from build123d import *

# Parameters (mm, degrees)
EXTRUDE_1_DEPTH     = 35
SKETCH_2_R          = 1.75
CUT_EXTRUDE_1_DEPTH = 40.39586793
SKETCH_3_W          = 0.8
SKETCH_3_H          = 10
EXTRUDE_2_DEPTH     = 35
SKETCH_4_R          = 2.7
CUT_EXTRUDE_2_DEPTH = 40.395868074


with BuildPart() as part:
    # Эскиз1 → Бобышка-Вытянуть1 (new body)
    with BuildSketch(Plane(origin=(0, 0, 0), x_dir=(1, 0, 0), z_dir=(0, 1, 0))):
        with BuildLine():
            Line((-4.558992206, 17.5), (0, 17.5))
            Line((0, 17.5), (0, -17.5))
            Line((0, -17.5), (-4.558992206, -17.5))
            ThreePointArc((-4.558992206, -17.5), (-3, 0), (-4.558992206, 17.5))
        make_face()
    extrude(amount=EXTRUDE_1_DEPTH)

    # Эскиз2 → Вырез-Вытянуть1 (cut, through all)
    with BuildSketch(Plane(origin=(0, 0, 0), x_dir=(0, 0, -1), z_dir=(1, 0, 0))):
        with Locations((-12, 25)):
            Circle(SKETCH_2_R)
        with Locations((12, 25)):
            Circle(SKETCH_2_R)
        with Locations((12, 10)):
            Circle(SKETCH_2_R)
        with Locations((-12, 10)):
            Circle(SKETCH_2_R)
    extrude(amount=-CUT_EXTRUDE_1_DEPTH, mode=Mode.SUBTRACT)

    # Эскиз3 → Бобышка-Вытянуть2 (add)
    with BuildSketch(Plane.XZ):
        with Locations((-3, 0)):
            Rectangle(SKETCH_3_W, SKETCH_3_H)
    extrude(amount=-EXTRUDE_2_DEPTH)

    # Эскиз4 → Вырез-Вытянуть2 (cut, through all)
    with BuildSketch(Plane(origin=(0, 0, 0), x_dir=(0, 0, -1), z_dir=(1, 0, 0))):
        with Locations((0, 17.5)):
            Circle(SKETCH_4_R)
    extrude(amount=-CUT_EXTRUDE_2_DEPTH, mode=Mode.SUBTRACT)


solid = part.part
Verification items for the finished model (mm, model axes). A direction names the side the tool comes from. Coordinates: 2 decimals unless noted, no trailing zeros. Loops run counter-clockwise (first coordinate to the right, second up) from the corner with the lowest first, then second, coordinate; pieces in that order, holes last. Notation, with made-up numbers: (84, 24) -> (120, 24) arc R22 cw to (120, 45) -> close; hole circle Ø2 at (75.5, 60.25). An arc over 180 degrees is marked (long way). Answer as CSV lines item,"result".
1) Cross-section at B-B, the plane y = 17.5. Record the cut outline in (x, z), then the cut area to 3 significant figures.
Found:
outline,"(-4.56, -17.5) -> (0, -17.5) -> (0, -2.7) -> (-3.4, -2.7) -> (-3.4, -5) -> (-3.13, -5) arc R99 cw to start; (-4.56, 17.5) arc R99 cw to (-3.13, 5) -> (-3.4, 5) -> (-3.4, 2.7) -> (0, 2.7) -> (0, 17.5) -> close"
area,"108 mm2"
2) Depth check by flat-ended pin: pin 1 (5 mm diameter, centred on y = 13, z = 2, fed in from -X); pin 2 (4.5 mm diameter, centred on y = 17.5, z = 0, fed in from +X); pin 3 (10 mm diameter, centred on y = 20, z = -9, fed in from -X). Enter the tip coordinate at first touch or a pass-through.
Found:
pin 1,"stops at x = -3.4"
pin 2,"passes through"
pin 3,"stops at x = -3.99"
3) Cross-section at A-A, the plane x = -1.8. Record the cut outline in (y, z), then the cut area to 3 significant figures.
Found:
outline,"(0, -17.5) -> (35, -17.5) -> (35, 17.5) -> (0, 17.5) -> close; hole circle Ø3.5 at (10, -12); hole circle Ø3.5 at (10, 12); hole circle Ø5.4 at (17.5, 0); hole circle Ø3.5 at (25, -12); hole circle Ø3.5 at (25, 12)"
area,"1,160 mm2"
4) Release check for a two-part mould opening along Y. For faces 1 (the flat face through (-2, 17, 17.5)), 2 (the cylindrical face through (-1.952, 25.526, -13.669)), 3 (the flat face through (-2, 35, 0)) record: +Y half, -Y half, draft (parallel to the pull), parting line (faces both ways), or undercut.
Found:
face 1,"draft"
face 2,"undercut"
face 3,"+Y half"
5) Cross-section at C-C, the plane z = 0. Record the cut outline in (x, y), then the cut area to 3 significant figures.
Found:
outline,"(-3.4, 0) -> (0, 0) -> (0, 14.8) -> (-3.4, 14.8) -> close; (-3.4, 20.2) -> (0, 20.2) -> (0, 35) -> (-3.4, 35) -> close"
area,"101 mm2"
6) Cross-section at D-D, the plane y = 10. Record the cut outline in (x, z).
Found:
outline,"(-4.56, -17.5) -> (0, -17.5) -> (0, -13.75) -> (-3.96, -13.75) arc R99 cw to start; (-4.56, 17.5) arc R99 cw to (-3.96, 13.75) -> (0, 13.75) -> (0, 17.5) -> close; (-3.53, -10.25) -> (0, -10.25) -> (0, 10.25) -> (-3.53, 10.25) arc R99 cw to (-3.13, 5) -> (-3.4, 5) -> (-3.4, -5) -> (-3.13, -5) arc R99 cw to start"
7) Thickness scan on L1, parallel to Y at x = -1.75, z = 12; L2, parallel to Z at x = -2.8, y = 10; L3, parallel to Y at x = -1.9, z = 13.5. Record the ranges inside material, lowest first. Write a range as from..to.
Found:
L1,"y = 0..8.25, 11.75..23.25, 26.75..35"
L2,"z = -17.5..-13.75, -10.25..10.25, 13.75..17.5"
L3,"y = 0..9.1, 10.9..24.1, 25.9..35"
8) Tool access check on faces 4 (the cylindrical face through (-3.654, 17.255, 11.36)), 5 (the cylindrical face through (-1.95, 25.08, 13.75)). Record the directions out of +Z, -Z, +X, -X, +Y, -Y that give a thin tool (end or side, any length) a straight path to the whole face; none if there is none.
Found:
face 4,"-X, +Y, -Y"
face 5,"+X, -X"
